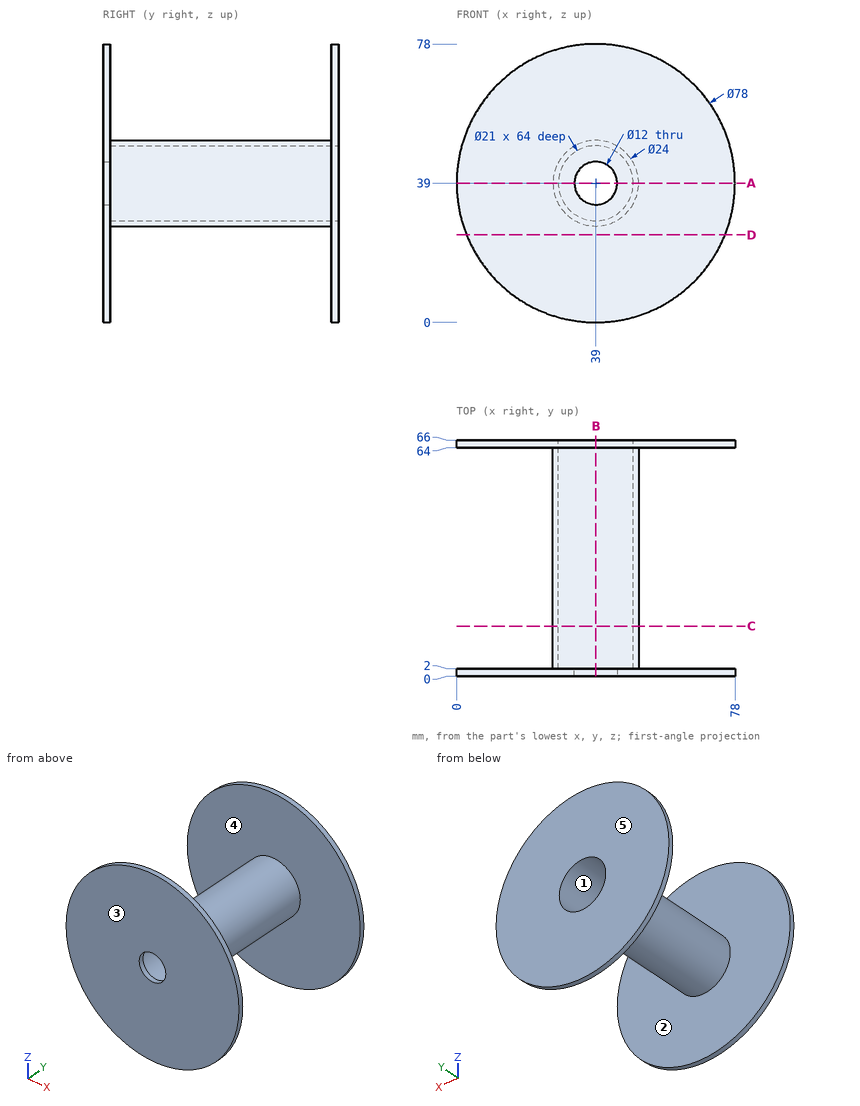
Job drawing, mm, ordinate dimensions from the low corner. One solid piece. A direction names the side the tool comes from. Coordinates: 2 decimals unless noted, no trailing zeros. Write each loop counter-clockwise with the first axis right and the second up, starting at its lowest first coordinate (ties: lowest second). Pieces come first, ordered by that corner, then holes. Notation, with made-up numbers: M -25,-18.5 L 32,-18.5 A28 cw 32,12.5 Z; hole C 51.5,52.5 d4. An arc over 180 degrees is marked long. Answer as a JSON object with one key per item and string values. Group by question number.
1) Saw through at B-B (x = 39). Write the cut outline in (y, z).
2) Saw through at C-C (y = 14). Write the cut outline in (x, z), plus the area to 3 significant figures.
3) Pin check, flat tips, straight feed: pin 1 Ø9.5 at (x, z) = (39, 39) entering from -Y; pin 2 Ø10.5 at (x, z) = (39.5, 43.5) entering from +Y; pin 3 Ø12.5 at (x, z) = (39, 39) entering from -Y; pin 4 Ø10 at (y, z) = (51, 47) entering from +X. Stop position of each tip, or through.
4) Mould opens along Y. For the marked faces 3, 4 and 5 say: +Y half, -Y half, draft (parallel to the pull), parting line (faces both ways), or undercut.
5) Wall check: line 1 (Y direction, x = 51, z = 63); line 2 (Z direction, x = 39, y = 50.5); line 3 (Z direction, x = 39, y = 0.75). Give the ranges that are in metal, low to high. Write a range as from..to.
6) Saw through at D-D (z = 24.5). Write the cut outline in (x, y).
7) Tool access for the marked faces 1 and 2: list every direction of +Z, -Z, +X, -X, +Y, -Y with a clear straight run to the whole face (end or side of a thin tool).
8) Saw through at A-A (z = 39). Write the cut outline in (x, y), plus the area to 3 significant figures.
Values follow:
{
 "1": {"outline": "M 0,0 L 2,0 L 2,27 L 64,27 L 64,0 L 66,0 L 66,28.5 L 2,28.5 L 2,33 L 0,33 Z; M 0,45 L 2,45 L 2,49.5 L 66,49.5 L 66,78 L 64,78 L 64,51 L 2,51 L 2,78 L 0,78 Z"},
 "2": {"outline": "C 39,39 d24; hole C 39,39 d21", "area": "106 mm2"},
 "3": {"pin 1": "passes through", "pin 2": "stops at y = 2", "pin 3": "stops at y = 0", "pin 4": "stops at x = 50.62"},
 "4": {"face 3": "-Y half", "face 4": "undercut", "face 5": "+Y half"},
 "5": {"line 1": "y = 0..2, 64..66", "line 2": "z = 27..28.5, 49.5..51", "line 3": "z = 0..33, 45..78"},
 "6": {"outline": "M 2.8,0 L 75.2,0 L 75.2,2 L 2.8,2 Z; M 2.8,64 L 75.2,64 L 75.2,66 L 2.8,66 Z"},
 "7": {"face 1": "+Y", "face 2": "none"},
 "8": {"outline": "M 0,0 L 33,0 L 33,2 L 28.5,2 L 28.5,66 L 0,66 L 0,64 L 27,64 L 27,2 L 0,2 Z; M 45,0 L 78,0 L 78,2 L 51,2 L 51,64 L 78,64 L 78,66 L 49.5,66 L 49.5,2 L 45,2 Z", "area": "432 mm2"}
}
